```python
from build123d import *

# Parameters (mm, degrees)
SKETCH1_R           = 5
BOSS_EXTRUDE1_DEPTH = 100
SKETCH2_W           = 5.740134486
SKETCH2_H           = 2.400249814
SKETCH2_W_2         = 4.427188802
CUT_EXTRUDE1_DEPTH  = 101
FILLET1_R           = 0.9


with BuildPart() as part:
    # Sketch1 → Boss-Extrude1 (new body)
    with BuildSketch(Plane(origin=(0, 0, 0), x_dir=(0, 0, -1), z_dir=(1, 0, 0))):
        Circle(SKETCH1_R)
    extrude(amount=BOSS_EXTRUDE1_DEPTH)

    # Sketch2 → Cut-Extrude1 (cut, through all)
    with BuildSketch(Plane(origin=(100, 0, 0), x_dir=(0, 0, -1), z_dir=(1, 0, 0))):
        with Locations((-2.870067243, 4.700124907)):
            Rectangle(SKETCH2_W, SKETCH2_H)
        with Locations((2.213594401, 4.700124907)):
            Rectangle(SKETCH2_W_2, SKETCH2_H)
    extrude(amount=-CUT_EXTRUDE1_DEPTH, mode=Mode.SUBTRACT)

    # Fillet1
    fillet1_edges = [part.edges().sort_by_distance(p)[0] for p in [
        (50, 3.5, -3.570714214),
        (50, 3.5, 3.570714214),
    ]]
    fillet(fillet1_edges, radius=FILLET1_R)


solid = part.part
```
The model under review builds one solid part; all positions refer to its coordinate system, in mm. Round coordinates to 2 decimals unless told otherwise and drop trailing zeros. Loops run counter-clockwise (first coordinate to the right, second up) from the corner with the lowest first, then second, coordinate; pieces in that order, holes last. Notation, with made-up numbers: (-26, -37) - (-7, -37) arc R16 cw to (-7, -10) - close; hole circle Ø2 at (2, 4). An arc over 180 degrees is marked (long way). Use a Markdown table: item, result. Add a question column.
Q1. Insertion check: pin 1 Ø1 at (x, y) = (46, -3) entering from -Z. The pin has a flat end and moves straight along its axis. Give the tip position at first contact, or say it passes through.
Q2. For probe 1 along Y at (x, z) = (87, 0.25); probe 2 along Z at (x, y) = (38.5, -0.25); probe 3 along Z at (x, y) = (25, -4), list the stretches that pass through material, from the lowest coordinate up.
Q3. Add section A-A (x = 45.5). State the section outline as (y, z) points, plus the area to 3 significant figures.
Q4. Add section B-B (y = -2.5). State the section outline as (x, z) points, plus the area to 3 significant figures.
Worked answers:
| question | item | result |
|---|---|---|
| 1 | pin 1 | z = -4.33 |
| 2 | probe 1 | -4.99 to 3.5 |
| 2 | probe 2 | -4.99 to 4.99 |
| 2 | probe 3 | -3 to 3 |
| 3 | outline | (3.17, -3.87) arc R0.9 ccw to (3.5, -3.17) - (3.5, 3.17) arc R0.9 ccw to (3.17, 3.87) arc R5 ccw (long way) to start |
| 3 | area | 71.1 mm² |
| 4 | outline | (0, -4.33) - (100, -4.33) - (100, 4.33) - (0, 4.33) - close |
| 4 | area | 866 mm² |
